The listing builds one solid part. Answer for the finished solid, in the listing's coordinates (mm). A direction names the side the tool comes from. Coordinates: 2 decimals unless noted, no trailing zeros. Order: outer loops, then holes, each group sorted by start corner. A loop starts at its lowest first (then second) coordinate and runs counter-clockwise, first axis right, second up. Notation, with made-up numbers: M 18.25,70.25 L 28.25,70.25 A23 ccw 28.25,90.25 Z; hole C -14,27.5 d8. An arc over 180 degrees is marked long. One line per item, written item: value. Start each with the question number.
Q1. The part is cut by section C-C on x = 5.75. Give the vertices of the cut face in (y, z).
Q2. Straight lines are drawn through the part: line 1 along Z through (x, y) = (0.5, -1.5); line 2 along X through (y, z) = (-0.75, 3.5); line 3 along Z through (x, y) = (4.5, -3.25). For each, find the intervals that lie inside material, in ascending order. Write a range as [from, to].
Q3. The part is cut by section D-D on z = -0.5. Give the vertices of the cut face in (x, y), then the cut area to 3 significant figures.
Q4. The part is cut by section A-A on y = -5.95. Give the vertices of the cut face in (x, z), then the cut area to 3 significant figures.
Q5. The part is cut by section B-B on z = 5.95. Give the vertices of the cut face in (x, y).
Q6. Each of these flat-tipped pins is pushed along its axis until it touches: pin 1 Ø2.5 at (y, z) = (-6, -3) entering from +X; pin 2 Ø1.5 at (y, z) = (-9.5, 3.5) entering from +X; pin 3 Ø0.8 at (x, z) = (1, -1.5) entering from -Y. Where does it stop, or does it pass through?
Q7. For faces 1 (the flat face through (0.2, -6, -2)), 2 (the flat face through (1, -9.3, -2)), 3 (the flat face through (3.8, -9, 3)), 4 (the flat face through (1, -2.6, -2)), determine the directions among +Z, -Z, +X, -X, +Y, -Y from which every point of the face is accessible in a straight line to the end or side of a thin tool.
Autodesk Fusion 360 part; units mm, degrees
sketch "Sketch1" plane through (0, 0, 0) normal (1, 0, 0) x (0, 1, 0)
  line L0 (0, 0) -> (-11.9, 0)
  line L1 (-11.9, 0) -> (-11.9, 11.9)
  line L2 (-11.9, 11.9) -> (0, 11.9)
  line L3 (0, 11.9) -> (0, 0)
  dimension "d1" = 11.9
  dimension "d2" = 11.9
extrude "Extrude1" add sketch "Sketch1" along normal blind 3.8
sketch "Sketch2" plane through (3.8, 0, 0) normal (1, 0, 0) x (0, 1, 0)
  line L0 (0, 11.9) -> (-11.9, 11.9)
  line L1 (-11.9, 11.9) -> (-11.9, 0)
  line L2 (-11.9, 0) -> (0, 0)
  line L3 (0, 0) -> (0, 11.9)
  line L4 (-5.95, 11.9) -> (-5.95, 0)
  line L5 (0, 5.95) -> (-11.9, 5.95)
  circle A0 centre (-5.95, 5.95) radius 3.35
  dimension "d5" = 6.7
extrude "Extrude2" add sketch "Sketch2" along normal blind 2.8 contours L4 L5 A0 | L4 L5 A0 | L4 L5 A0 | L4 L5 A0
sketch "Sketch3" plane through (0, 0, 0) normal (0, 0, -1) x (1, 0, 0)
  line L0 (0, 11.9) -> (0, 0)
  line L1 (0, 0) -> (3.8, 0)
  line L2 (3.8, 0) -> (3.8, 11.9)
  line L3 (3.8, 11.9) -> (0, 11.9)
  line L4 (0.2, 9.3) -> (1.8, 9.3)
  line L5 (1.8, 9.3) -> (1.8, 2.6)
  line L6 (1.8, 2.6) -> (0.2, 2.6)
  line L7 (0.2, 2.6) -> (0.2, 9.3)
  dimension "d8" = 2.6
  dimension "d10" = 2.6
  dimension "d11" = 0.2
  dimension "d12" = 2
extrude "Extrude3" add sketch "Sketch3" along normal blind 4.6 contours L4 L5 L6 L7
equation "d10 = d8"
Output:
1. outline: C -5.95,5.95 d6.7
2. line 1: z = [0, 11.9]
2. line 2: x = [0, 3.8]
2. line 3: z = [3.97, 7.93]
3. outline: M 0.2,-9.3 L 1.8,-9.3 L 1.8,-2.6 L 0.2,-2.6 Z
3. area: 10.7 mm^2
4. outline: M 0,0 L 0.2,0 L 0.2,-4.6 L 1.8,-4.6 L 1.8,0 L 3.8,0 L 3.8,2.6 L 6.6,2.6 L 6.6,9.3 L 3.8,9.3 L 3.8,11.9 L 0,11.9 Z
4. area: 71.3 mm^2
5. outline: M 0,-11.9 L 3.8,-11.9 L 3.8,-9.3 L 6.6,-9.3 L 6.6,-2.6 L 3.8,-2.6 L 3.8,0 L 0,0 Z
6. pin 1: stops at x = 1.8
6. pin 2: stops at x = 3.8
6. pin 3: stops at y = -9.3
7. face 1: -Z, -X, +Y, -Y
7. face 2: -Z, +X, -X, -Y
7. face 3: +X
7. face 4: -Z, +X, -X, +Y
